```python
from build123d import *

# Parameters (mm, degrees)
F1_DEPTH = 25.4
F2_W     = 0.254
F2_H     = 25.4
F4_W     = 0.254
F4_H     = 25.4


with BuildPart() as f1:
    # F0 (on Top) → F1 (new body)
    with BuildSketch(Plane.XY):
        with BuildLine():
            Line((-3.175, 0), (0, 0))
            Line((0, 0), (0, 25.4))
            ThreePointArc((0, 25.4), (25.4, 50.8), (50.8, 25.4))
            Line((50.8, 25.4), (50.8, 0))
            Line((50.8, 0), (53.975, 0))
            Line((53.975, 0), (53.975, 25.4))
            ThreePointArc((53.975, 25.4), (25.4, 53.975), (-3.175, 25.4))
            Line((-3.175, 25.4), (-3.175, 0))
        make_face()
    extrude(amount=F1_DEPTH)

    # F3: sweep along a path in F3_path
    with BuildLine(Plane(origin=(-3.175, 0, 25.4), x_dir=(0, 0, -1), z_dir=(0, 1, 0))) as f3_path:
        Line((0, 0), (25.4, 0))
        Line((25.4, 0), (25.4, -3.175))
        Line((25.4, -3.175), (0, -3.175))
        Line((0, -3.175), (0, 0))
    # F2 (on face) → F3 (sweep, cut)
    with BuildSketch(Plane.XY.offset(25.4)):
        with Locations((-3.048, 12.7)):
            Rectangle(F2_W, F2_H)
    sweep(path=f3_path.line, transition=Transition.RIGHT, mode=Mode.SUBTRACT)

    # F5: sweep along a path in F5_path
    with BuildLine(Plane(origin=(50.8, 0, 0), x_dir=(0, 0, 1), z_dir=(0, -1, 0))) as f5_path:
        Line((0, 0), (25.4, 0))
        Line((25.4, 0), (25.4, -3.175))
        Line((25.4, -3.175), (0, -3.175))
        Line((0, -3.175), (0, 0))
    # F4 (on face) → F5 (sweep, cut)
    with BuildSketch(Plane.XY.offset(25.4)):
        with Locations((50.927, 12.7)):
            Rectangle(F4_W, F4_H)
    sweep(path=f5_path.line, transition=Transition.RIGHT, mode=Mode.SUBTRACT)


solid = f1.part
```
CAD build for the part. Positions are in the model's coordinates, mm. A direction names the side the tool comes from. Give positions to 0.01 mm unless a question says otherwise; leave off trailing zeros. Loops run counter-clockwise (first coordinate to the right, second up) from the corner with the lowest first, then second, coordinate; pieces in that order, holes last. Notation, with made-up numbers: (11, -3.5) -> (22, -3.5) arc R32 cw to (22, 24.5) -> close; hole circle Ø1 at (-5, -18). An arc over 180 degrees is marked (long way). Use a Markdown table: item, result.
1. Which spindle directions (+Z, -Z, +X, -X, +Y, -Y) get a long thin tool onto all of the face, cutting with end or side? Do faces 1 (the flat face through (51.054, 13, 13)), 2 (the flat face through (52, 13, 0.254)), 3 (the flat face through (53.721, 13, 13)), 4 (the flat face through (52, 13, 25.146)). Say none if no direction does.
Check result:
| item | result |
|---|---|
| face 1 | +Z, -Z, -Y |
| face 2 | -Z, +X, -X, -Y |
| face 3 | +Z, -Z, +X, -Y |
| face 4 | +Z, +X, -X, -Y |
2. Slice it at A-A (y = 22). List the corners of the cut face in (x, z).
Check result:
| item | result |
|---|---|
| outline | (-2.92, 0.25) -> (-0.25, 0.25) -> (-0.25, 25.15) -> (-2.92, 25.15) -> close; (51.05, 0.25) -> (53.72, 0.25) -> (53.72, 25.15) -> (51.05, 25.15) -> close |
3. Wall check: L1, parallel to X at y = 13, z = 23; L2, parallel to X at y = 25.5, z = 18; L3, parallel to Y at x = 41, z = 23. Give the ranges that are in metal, low to high. Write a range as [from, to].
Check result:
| item | result |
|---|---|
| L1 | x = [-2.92, -0.25], [51.05, 53.72] |
| L2 | x = [-3.17, 0], [50.8, 53.97] |
| L3 | y = [45.44, 49.34] |
4. Slice it at D-D (x = 25.4). List the corners of the cut face in (y, z) (3 decimals), plus the area to 3 significant figures.
Check result:
| item | result |
|---|---|
| outline | (50.8, 0) -> (53.975, 0) -> (53.975, 25.4) -> (50.8, 25.4) -> close |
| area | 80.6 mm^2 |
5. Flat gauge pins, fed straight in: pin 1 (12 mm diameter, centred on y = 6, z = 9, fed in from +X); pin 2 (12 mm diameter, centred on y = 46.5, z = 10, fed in from +X); pin 3 (10 mm diameter, centred on x = 10.5, z = 6, fed in from -Y). Where does each tip first touch, or does it go through?
Check result:
| item | result |
|---|---|
| pin 1 | stops at x = 53.72 |
| pin 2 | stops at x = 49.66 |
| pin 3 | stops at y = 41.18 |
6. Mould opens along X. For faces 5 (the flat face through (-2, 13, 0.254)), 6 (the flat face through (-0.254, 13, 13)), 7 (the flat face through (-2.921, 13, 13)) say: pulls with the +X half, pulls with the -X half, needs draft (parallel to the pull), parting line crosses it, or undercut.
Check result:
| item | result |
|---|---|
| face 5 | needs draft |
| face 6 | undercut |
| face 7 | pulls with the -X half |
7. Slice it at C-C (y = 39). List the corners of the cut face in (x, z), plus the area to 3 significant figures.
Check result:
| item | result |
|---|---|
| outline | (0.27, 0) -> (3.95, 0) -> (3.95, 25.4) -> (0.27, 25.4) -> close; (46.85, 0) -> (50.53, 0) -> (50.53, 25.4) -> (46.85, 25.4) -> close |
| area | 187 mm^2 |
8. Slice it at B-B (z = 22). List the corners of the cut face in (x, y) (3 decimals).
Check result:
| item | result |
|---|---|
| outline | (-3.175, 25.4) -> (-2.921, 25.4) -> (-2.921, 0) -> (-0.254, 0) -> (-0.254, 25.4) -> (0, 25.4) arc R25.4 cw to (50.8, 25.4) -> (51.054, 25.4) -> (51.054, 0) -> (53.721, 0) -> (53.721, 25.4) -> (53.975, 25.4) arc R28.575 ccw to start |
